Autodesk Inventor part; units mm, degrees
ref_plane "Work Plane1" through (0, 0, 7) normal (0, 0, 1) x (1, 0, 0)
ref_plane "YZ Plane" through (0, 0, 0) normal (1, 0, 0) x (0, 1, 0)
ref_plane "XZ Plane" through (0, 0, 0) normal (0, 1, 0) x (-1, 0, 0)
sketch "Sketch1" plane through (0, 0, 0) normal (0, 0, 1) x (1, 0, 0)
  circle A0 centre (0, 0) radius 13.3333
  dimension "d0" = 26.6667
extrude "Extrusion1" add sketch "Sketch1" along normal blind 2
sketch "Sketch2" plane through (0, 0, 2) normal (0, 0, 1) x (1, 0, 0)
  circle A0 centre (0, 0) radius 2.5
  dimension "d3" = 5
extrude "Extrusion2" add sketch "Sketch2" along normal blind 7
ref_plane "Work Plane1" through (0, 0, 7) normal (0, 0, 1) x (1, 0, 0)
sketch "Sketch5" plane through (0, 0, 7) normal (0, 0, 1) x (1, 0, 0)
  circle A0 centre (0, 0) radius 2.5
  circle A1 centre (0, 0) radius 3.5
  dimension "d18" = 1
extrude "Extrusion7" add sketch "Sketch5" against normal blind 1
sketch "Sketch6" plane through (0, 0, 0) normal (0, 0, -1) x (-1, 0, 0)
  circle A0 centre (0, 0) radius 13.3333
  circle A1 centre (0, 0) radius 2.5
  line L0 (-2.5, 0) -> (2.5, 0)
  line L1 (2.5, 0) -> (2.5, -24.6522)
  line L2 (2.5, -24.6522) -> (-2.5, -24.6522)
  line L3 (-2.5, -24.6522) -> (-2.5, 0)
  circle A2 centre (0, 0) radius 2.5
  point P0 (2.5, 0)
  dimension "d23" = 5
  dimension "d24" = 5
  dimension "d25" = 24.6522
extrude "Extrusion8" add sketch "Sketch6" along normal blind 2.5 contours L3 A1 L1 A0 | A0 L1 L2 L3 | L0 A1 | A1 L0 picked at (-0.1004, -9.6986)
sketch "Sketch8" plane through (0, 0, 9) normal (0, 0, 1) x (1, 0, 0)
  circle A0 centre (0, 0) radius 2.5
extrude "Extrusion10" add sketch "Sketch8" along normal blind 3
equation "\"d0\" = OG_gearDiameter"
equation "\"d1\" = OG_gearThickness"
equation "\"d3\" = OG_shaftDiameter"
equation "\"d4\" = OG_shaftLength"
equation "\"d18\" = OG_skirtOffset"
equation "\"d19\" = OG_skirtThickness"
equation "\"Wheel_Related_W_\" = 0"
equation "\"W_innerDepth\" = 4"
equation "\"W_wallThickness\" = 2"
equation "\"W_holesClearance\" = 0.3"
equation "\"W_outerGearHoleDiameter\" = 5.3"
equation "\"W_innerGearHoleDiameter\" = 10.1"
equation "\"TempSpotReserved7\" = 0"
equation "\"TempSpotReserved8\" = 0"
equation "\"TempSpotReserved9\" = 0"
equation "\"TempSpotReserved10\" = 0"
equation "\"TempSpotReserved11\" = 0"
equation "\"TempSpotReserved12\" = 0"
equation "\"TempSpotReserved13\" = 0"
equation "\"TempSpotReserved14\" = 0"
equation "\"TempSpotReserved15\" = 0"
equation "\"TempSpotReserved16\" = 0"
equation "\"TempSpotReserved17\" = 0"
equation "\"TempSpotReserved18\" = 0"
equation "\"TempSpotReserved19\" = 0"
equation "\"TempSpotReserved20\" = 0"
equation "\"Inner_Gear_Related_IG_\" = 0"
equation "\"IG_shaftDiameter\" = 7.5"
equation "\"IG_shaftLength\" = 15"
equation "\"IG_gearThickness\" = 2"
equation "\"TempSpotReserved25\" = 0"
equation "\"TempSpotReserved26\" = 0"
equation "\"TempSpotReserved27\" = 0"
equation "\"TempSpotReserved28\" = 0"
equation "\"TempSpotReserved29\" = 0"
equation "\"TempSpotReserved30\" = 0"
equation "\"TempSpotReserved31\" = 0"
equation "\"TempSpotReserved32\" = 0"
equation "\"TempSpotReserved33\" = 0"
equation "\"TempSpotReserved34\" = 0"
equation "\"TempSpotReserved35\" = 0"
equation "\"TempSpotReserved36\" = 0"
equation "\"TempSpotReserved37\" = 0"
equation "\"TempSpotReserved38\" = 0"
equation "\"TempSpotReserved39\" = 0"
equation "\"TempSpotReserved40\" = 0"
equation "\"Outer_Gear_Related_OG_\" = 0"
equation "\"OG_distanceFromCenter\" = 23.33333"
equation "\"OG_shaftDiameter\" = 5"
equation "\"OG_gearDiameter\" = 26.66667"
equation "\"OG_shaftLength\" = 7"
equation "\"OG_gearThickness\" = 2"
equation "\"TempSpotReserved47\" = 0"
equation "\"TempSpotReserved48\" = 0"
equation "\"TempSpotReserved49\" = 0"
equation "\"TempSpotReserved50\" = 0"
equation "\"TempSpotReserved51\" = 0"
equation "\"TempSpotReserved52\" = 0"
equation "\"TempSpotReserved53\" = 0"
equation "\"TempSpotReserved54\" = 0"
equation "\"TempSpotReserved55\" = 0"
equation "\"TempSpotReserved56\" = 0"
equation "\"TempSpotReserved57\" = 0"
equation "\"TempSpotReserved58\" = 0"
equation "\"TempSpotReserved59\" = 0"
equation "\"TempSpotReserved60\" = 0"
equation "\"Leg_Extensions_Related_LE_\" = 0"
equation "\"LE_baseDiameter\" = 5"
equation "\"LE_maxLength\" = 24.6522"
equation "\"LE_thickness\" = 2.5"
equation "\"IG_ratioToOuterGear\" = 0.75"
equation "\"B_bearingThickness\" = 1"
equation "\"TempSpotReserved43\" = 0"
equation "\"TempSpotReserved45\" = 0"
equation "\"Thisisatest\" = 25.4"
equation "\"TempSpotReserved46\" = 0"
equation "\"TempSpotReserved44\" = 0"
equation "\"LE_offsetAboveOuterGear\" = 0"
equation "\"Bearing_Related_B_\" = 0"
equation "\"TempSpotReserved42\" = 0"
equation "\"d17\" = -W_wallThickness"
equation "\"OG_skirtOffset\" = 1"
equation "\"OG_skirtThickness\" = 1"
equation "\"IG_skirtThickness\" = 2"
equation "\"IG_extentionLength\" = 18.33333"
equation "\"IG_extentionThickness\" = 3"
equation "\"IG_slitWidth\" = 4"
equation "\"IG_slitlength\" = 8"
equation "\"IG_slitDistanceFromCenterHole\" = 8"
equation "\"IG_slitClearance\" = 0.2"
equation "\"Reserved_10\" = 0"
equation "\"Reserved_9\" = 0"
equation "\"Reserved_11\" = 0"
equation "\"Reserved_12\" = 0"
equation "\"Reserved_8\" = 0"
equation "\"Reserved_7\" = 0"
equation "\"Reserved_26\" = 0"
equation "\"Reserved_20\" = 0"
equation "\"Reserved_22\" = 0"
equation "\"Reserved_23\" = 0"
equation "\"Reserved_25\" = 0"
equation "\"Reserved_24\" = 0"
equation "\"Reserved_21\" = 0"
equation "\"Reserved_19\" = 0"
equation "\"Reserved_27\" = 0"
equation "\"Reserved_14\" = 0"
equation "\"Reserved_15\" = 0"
equation "\"Reserved_16\" = 0"
equation "\"Reserved_13\" = 0"
equation "\"Reserved_17\" = 0"
equation "\"Reserved_18\" = 0"
equation "\"Bearing_Related_BR_\" = 0"
equation "\"BR_bearingThickness\" = 1"
equation "\"Block_Related_BL_\" = 0"
equation "\"BL_width\" = 3.8"
equation "\"BL_length\" = 7.8"
equation "\"W_filletRadius\" = 0.25"
equation "\"W_extrutsionTaperAngle\" = 2deg"
equation "\"OG_protrudeDistance\" = 3"
properties part number "outerGear"
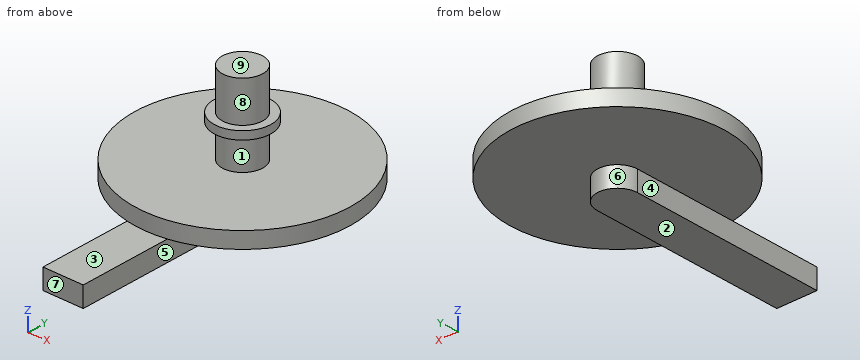
Read the model definition and answer for the solid it produces. Units are mm, in the model's axes. Face numbers are marked on the shaded views. A direction names the side the tool comes from. Coordinates: 2 decimals unless noted, no trailing zeros. Loops run counter-clockwise (first coordinate to the right, second up) from the corner with the lowest first, then second, coordinate; pieces in that order, holes last. Notation, with made-up numbers: (-8, 15.5) - (0, 15.5) arc R31 ccw to (0, 40.5) - close; hole circle Ø4 at (0, -22). An arc over 180 degrees is marked (long way). Answer in a Markdown table with one row per item.
1. Which of the six approach directions +Z, -Z, +X, -X, +Y, -Y give full straight-line access (tool end or side, diameter ignored) to the marked faces 5, 6, 7, 8 and 9?
Conclusion:
| item | result |
|---|---|
| face 5 | -Z, +X, +Y, -Y |
| face 6 | -Z, +Y |
| face 7 | +Z, -Z, +X, -X, -Y |
| face 8 | +Z |
| face 9 | +Z, +X, -X, +Y, -Y |
2. Find section D-D, the plane x = -9.75. Write down the section's boundary in (y, z).
Conclusion:
| item | result |
|---|---|
| outline | (-9.09, 0) - (9.09, 0) - (9.09, 2) - (-9.09, 2) - close |
3. Find section C-C, the plane z = 3.5. Write down the section's boundary in (x, y).
Conclusion:
| item | result |
|---|---|
| outline | circle Ø5 at (0, 0) |
4. Given pin 1 (1.2 mm diameter, centred on y = -16.5, z = -1.5, fed in from +X); pin 2 (5.5 mm diameter, centred on x = 1, y = -18, fed in from +Z); pin 3 (1.2 mm diameter, centred on y = -11.5, z = -2, fed in from -X), each flat-ended and moving along its own axis, determine where each tip first touches the part or whether it passes through.
Conclusion:
| item | result |
|---|---|
| pin 1 | stops at x = 2.5 |
| pin 2 | stops at z = 0 |
| pin 3 | stops at x = -2.5 |
5. Determine the mould class of the marked faces 1, 2, 3 and 4 for opening direction Z: +Z half, -Z half, draft (parallel to the pull), parting line (faces both ways), or undercut.
Conclusion:
| item | result |
|---|---|
| face 1 | undercut |
| face 2 | -Z half |
| face 3 | +Z half |
| face 4 | draft |
6. Find section B-B, the plane y = -21. Write down the section's boundary in (x, z).
Conclusion:
| item | result |
|---|---|
| outline | (-2.5, -2.5) - (2.5, -2.5) - (2.5, 0) - (-2.5, 0) - close |
7. Straight lines are drawn through the part: line 1 (Z direction, x = 3.75, y = 7); line 2 (Z direction, x = 3, y = -1.5); line 3 (Z direction, x = 1.5, y = -4.5). For each, find the intervals that lie inside material, in ascending order.
Conclusion:
| item | result |
|---|---|
| line 1 | z = 0 to 2 |
| line 2 | z = 0 to 2, 6 to 7 |
| line 3 | z = -2.5 to 2 |
8. Find section A-A, the plane x = 0. Write down the section's boundary in (y, z).
Conclusion:
| item | result |
|---|---|
| outline | (-24.65, -2.5) - (2.5, -2.5) - (2.5, 0) - (13.33, 0) - (13.33, 2) - (2.5, 2) - (2.5, 6) - (3.5, 6) - (3.5, 7) - (2.5, 7) - (2.5, 12) - (-2.5, 12) - (-2.5, 7) - (-3.5, 7) - (-3.5, 6) - (-2.5, 6) - (-2.5, 2) - (-13.33, 2) - (-13.33, 0) - (-24.65, 0) - close |
